Source: CAD feature listing. Evaluate the final solid. Frame: model axes, mm. A direction names the side the tool comes from. Coordinates: 2 decimals unless noted, no trailing zeros. Loops run counter-clockwise (first coordinate to the right, second up) from the corner with the lowest first, then second, coordinate; pieces in that order, holes last.
Autodesk Fusion 360 part; units mm, degrees
sketch "Sketch1" plane through (0, 0, 0) normal (0, 1, 0) x (1, 0, 0)
  line L0 (0, -1.5) -> (0, 14)
  line L1 (0, 14) -> (0.75, 14)
  line L2 (0.75, 14) -> (1.25, 13.5)
  line L3 (1.25, 13.5) -> (1.25, 0)
  line L4 (1.25, 0) -> (2.25, 0)
  line L5 (2.25, 0) -> (2.25, -0.4)
  line L6 (0, -1.5) -> (1, -1.5)
  arc A0 (1, -1.5) -> (2.25, -0.4) centre (0, 0.8966) ccw
  dimension "d1" = 14
  dimension "d2" = 1.5
  dimension "d3" = 1
  dimension "d4" = 0.4
  dimension "d5" = 2.25
  dimension "d6" = 1.25
  dimension "d7" = 45
  dimension "d8" = 0.5
revolve "Revolve1" add sketch "Sketch1" angle 360 about axis through (0, 0, 1.5) along (0, 0, -1)
sketch "Sketch2" plane through (0, 0, 1.5) normal (0, 0, 1) x (-1, 0, 0)
  circle A0 centre (0, 0) radius 1
  line L0 (-0.75, -0.433) -> (0, -0.866)
  line L1 (0, -0.866) -> (0.75, -0.433)
  line L2 (0.75, -0.433) -> (0.75, 0.433)
  line L3 (0.75, 0.433) -> (0, 0.866)
  line L4 (0, 0.866) -> (-0.75, 0.433)
  line L5 (-0.75, 0.433) -> (-0.75, -0.433)
  dimension "d10" = 1.5
extrude "Extrude1" cut sketch "Sketch2" against normal up to surface (2 mm away) contours L0 L1 L2 L3 L4 L5
equation "d5 = ( 4.5 / 2 ) * 1 mm"
equation "d6 = ( 2.5 / 2 ) * 1 mm"

Autodesk Fusion 360 part; units mm, degrees
sketch "Sketch1" plane through (0, 0, 0) normal (0, 1, 0) x (1, 0, 0)
  line L0 (0, -1.5) -> (0, 4)
  line L1 (0, 4) -> (0.75, 4)
  line L2 (0.75, 4) -> (1.25, 3.5)
  line L3 (1.25, 3.5) -> (1.25, 0)
  line L4 (1.25, 0) -> (2.25, 0)
  line L5 (2.25, 0) -> (2.25, -0.4)
  line L6 (0, -1.5) -> (1, -1.5)
  arc A0 (1, -1.5) -> (2.25, -0.4) centre (0, 0.8966) ccw
  dimension "d1" = 4
  dimension "d2" = 1.5
  dimension "d3" = 1
  dimension "d4" = 0.4
  dimension "d5" = 2.25
  dimension "d6" = 1.25
  dimension "d7" = 45
  dimension "d8" = 0.5
revolve "Revolve1" add sketch "Sketch1" angle 360 about axis through (0, 0, 1.5) along (0, 0, -1)
sketch "Sketch2" plane through (0, 0, 1.5) normal (0, 0, 1) x (-1, 0, 0)
  circle A0 centre (0, 0) radius 1
  line L0 (-0.75, -0.433) -> (0, -0.866)
  line L1 (0, -0.866) -> (0.75, -0.433)
  line L2 (0.75, -0.433) -> (0.75, 0.433)
  line L3 (0.75, 0.433) -> (0, 0.866)
  line L4 (0, 0.866) -> (-0.75, 0.433)
  line L5 (-0.75, 0.433) -> (-0.75, -0.433)
  dimension "d10" = 1.5
extrude "Extrude1" cut sketch "Sketch2" against normal up to surface (2 mm away) contours L0 L1 L2 L3 L4 L5
equation "d5 = ( 4.5 / 2 ) * 1 mm"
equation "d6 = ( 2.5 / 2 ) * 1 mm"

Autodesk Fusion 360 part; units mm, degrees
sketch "Sketch1" plane through (0, 0, 0) normal (0, 1, 0) x (1, 0, 0)
  line L0 (0, -2) -> (0, 12)
  line L1 (0, 12) -> (0.45, 12)
  line L2 (0.45, 12) -> (0.95, 11.5)
  line L3 (0.95, 11.5) -> (0.95, 0)
  line L4 (0.95, 0) -> (1.9, 0)
  line L5 (1.9, 0) -> (1.9, -2)
  line L6 (1.9, -2) -> (0, -2)
  dimension "d1" = 12
  dimension "d2" = 45
  dimension "d3" = 0.5
  dimension "d4" = 0.95
  dimension "d5" = 2
  dimension "d6" = 1.9
revolve "Revolve1" add sketch "Sketch1" angle 360 about axis through (0, 0, 2) along (0, 0, -1)
sketch "Sketch2" plane through (0, 0, 2) normal (0, 0, 1) x (-1, 0, 0)
  circle A0 centre (0, 0) radius 1.9
  line L0 (-0.75, -0.433) -> (0, -0.866)
  line L1 (0, -0.866) -> (0.75, -0.433)
  line L2 (0.75, -0.433) -> (0.75, 0.433)
  line L3 (0.75, 0.433) -> (0, 0.866)
  line L4 (0, 0.866) -> (-0.75, 0.433)
  line L5 (-0.75, 0.433) -> (-0.75, -0.433)
  dimension "d8" = 1.5
extrude "Extrude1" cut sketch "Sketch2" against normal blind 1 contours L0 L1 L2 L3 L4 L5
equation "d4 = ( 1.9 / 2 ) * 1 mm"
equation "d6 = ( 3.8 / 2 ) * 1 mm"
Q1. Section query A-A on y = 0. Return the cut outline in (x, z), then the cut area to 4 significant figures.
Q2. Section query B-B on z = -0.5. Return the cut outline in (x, y).
Q3. Reachability of faces 4 (the cylindrical face through (-1.9, 0.08, 1.01)), 5 (the flat face through (-0.75, 0, 1.5)) from +Z, -Z, +X, -X, +Y, -Y: full face, straight path, thin tool, end or side. Return the list, or none.
Q4. Section query C-C on y = -1.6. Return the cut outline in (x, z), then the cut area to 3 significant figures.
Q5. Draft query along Y for faces 1 (the flat face through (1, 1, 0)), 2 (the cylindrical face through (-0.95, 0.04, -5.67)), 3 (the flat face through (0, 0, 1)). Return one class per face: released by +Y, released by -Y, zero draft, split by the parting line, or undercut.
Q6. Material intervals for line 1 along Z through (x, y) = (0.85, 1.5); line 2 along X through (y, z) = (0.4, -6.75); line 3 along Y through (x, z) = (0.1, -5.75), sorted ascending.
Q7. First-contact query: pin 1 Ø1.5 at (y, z) = (0.5, -10) entering from -X; pin 2 Ø1.6 at (x, y) = (0, 0) entering from +Z. Flat tips, straight axial feed; report the tip coordinate or a pass-through.
Resolved:
1. outline: (-1.9, 0) - (-0.95, 0) - (-0.95, -11.5) - (-0.45, -12) - (0.45, -12) - (0.95, -11.5) - (0.95, 0) - (1.9, 0) - (1.9, 2) - (0.75, 2) - (0.75, 1) - (-0.75, 1) - (-0.75, 2) - (-1.9, 2) - close
1. area: 28.65 mm2
2. outline: circle Ø1.9 at (0, 0)
3. face 4: +Z, -Z
3. face 5: +Z
4. outline: (-1.02, 0) - (1.02, 0) - (1.02, 2) - (-1.02, 2) - close
4. area: 4.10 mm2
5. face 1: zero draft
5. face 2: split by the parting line
5. face 3: undercut
6. line 1: z = 0 to 2
6. line 2: x = -0.86 to 0.86
6. line 3: y = -0.94 to 0.94
7. pin 1: stops at x = -0.95
7. pin 2: stops at z = 2
